Design review of the part built by this model. Coordinates are the model's own, in mm. A direction names the side the tool comes from. Give positions to 0.01 mm unless a question says otherwise; leave off trailing zeros. Order: outer loops, then holes, each group sorted by start corner. A loop starts at its lowest first (then second) coordinate and runs counter-clockwise, first axis right, second up. Notation, with made-up numbers: (83, 64.25) -> (127, 64.25) arc R8 ccw to (127, 75.25) -> close; hole circle Ø4 at (66, 2.25). An arc over 180 degrees is marked (long way). Answer in a Markdown table with one row per item. Add a question column.
```python
from build123d import *

# Parameters (mm, degrees)
BOSS_EXTRUDE1_DEPTH                                = 5.9944
FILLET1_R                                          = 1.5875
CSK_FOR_10_FLAT_HEAD_MACHINE_SCREW_100_D           = 5.1054
CSK_FOR_10_FLAT_HEAD_MACHINE_SCREW_100_CSINK_D     = 9.779
CSK_FOR_10_FLAT_HEAD_MACHINE_SCREW_100_CSINK_ANGLE = 100


with BuildPart() as part:
    # Sketch1 → Boss-Extrude1 (new body)
    with BuildSketch(Plane(origin=(0, 0, 0), x_dir=(1, 0, 0), z_dir=(0, 1, 0))):
        with BuildLine():
            Line((-35.898566824, -38.1), (35.898566824, -38.1))
            ThreePointArc((35.898566824, -38.1), (45.716712095, -35.375027517), (52.726020022, -27.9796875))
            ThreePointArc((52.726020022, -27.9796875), (59.69, 0), (52.726020022, 27.9796875))
            ThreePointArc((52.726020022, 27.9796875), (45.716712095, 35.375027517), (35.898566824, 38.1))
            Line((35.898566824, 38.1), (-35.898566824, 38.1))
            ThreePointArc((-35.898566824, 38.1), (-45.716712095, 35.375027517), (-52.726020022, 27.9796875))
            ThreePointArc((-52.726020022, 27.9796875), (-59.69, 0), (-52.726020022, -27.9796875))
            ThreePointArc((-52.726020022, -27.9796875), (-45.716712095, -35.375027517), (-35.898566824, -38.1))
        make_face()
    extrude(amount=BOSS_EXTRUDE1_DEPTH)

    # Sketch3 → Revolve1 (revolve)
    with BuildSketch(Plane.XY, mode=Mode.PRIVATE) as revolve1_sk:
        with BuildLine():
            Line((-29.9974, 5.9944), (0, 5.9944))
            Line((0, 5.9944), (0, 17.6022))
            ThreePointArc((0, 17.6022), (-11.253106327, 17.031245116), (-22.39063481, 15.324244597))
            ThreePointArc((-22.39063481, 15.324244597), (-27.854703555, 12.013305151), (-29.9974, 5.9944))
        make_face()
    revolve(revolve1_sk.sketch.rotate(Axis((0, 17.6022, 0), (0, -1, 0)), 180), axis=Axis((0, 17.6022, 0), (0, -1, 0)))

    # Fillet1
    fillet1_edges = [part.edges().sort_by_distance(p)[0] for p in [
        (-29.9974, 5.9944, 0),
    ]]
    fillet(fillet1_edges, radius=FILLET1_R)

    # CSK for #10 Flat Head Machine Screw (100)1 (through all)
    with Locations(Plane(origin=(0, 5.9944, 0), x_dir=(-1, 0, 0), z_dir=(0, 1, 0))):
        with Locations((41.91, -20.32), (41.91, 20.32), (-41.91, -20.32), (-41.91, 20.32)):
            CounterSinkHole(CSK_FOR_10_FLAT_HEAD_MACHINE_SCREW_100_D / 2, CSK_FOR_10_FLAT_HEAD_MACHINE_SCREW_100_CSINK_D / 2, counter_sink_angle=CSK_FOR_10_FLAT_HEAD_MACHINE_SCREW_100_CSINK_ANGLE)


solid = part.part
```
1) Add section C-C, the plane x = -34.5. Write out the cut boundary in (y, z), and give its area (3 significant figures).
2) Mouldability with a two-part tool opening along X and no side actions: class faces 3 (the face through (-44.03, 4.13, 18.7)), 4 (the face through (1, 3, -38.1)), 5 (the face through (45.84, 2.96, -35.3)) as +X half, -X half, draft (parallel to the pull), parting line (faces both ways), or undercut.
3) For L1, parallel to Z at x = -41.91, y = 3.15; L2, parallel to X at y = 2.7, z = -20.32; L3, parallel to Y at x = -24, z = 21, list the stretches that pass through material, from the lowest coordinate up.
4) Add section B-B, the plane z = 20.32. Give the number of separate pieces and of enclosed holes in the cut face, and give its area (3 significant figures).
5) Machinability: for faces 1 (the face through (59.69, 2.96, 0.41)), 2 (the face through (-27.4, 5.994, 16.4)), which of the approach directions +Z, -Z, +X, -X, +Y, -Y give a long, thin tool a straight path to every point of the face, cutting with its end or side? Answer none if there is none.
6) Add section A-A, the plane x = 41.91. Write out the cut boundary in (y, z).
7) Clearance check with flat-ended pins moving along their axes: P1, Ø3, axis at x = -41.91, z = -20.32, coming from the -Y side; P2, Ø1, axis at y = 13.5, z = -2.5, coming from the -X side; P3, Ø4, axis at y = 2, z = 2.5, coming from the -X side; P4, Ø4, axis at x = 16, y = 12, coming from the +Z side. State where each tip first meets the part, or that it passes through.
Verdict:
| question | item | result |
|---|---|---|
| 1 | outline | (0, -38.1) -> (5.99, -38.1) -> (5.99, 38.1) -> (0, 38.1) -> close |
| 1 | area | 457 mm2 |
| 2 | face 3 | undercut |
| 2 | face 4 | draft |
| 2 | face 5 | +X half |
| 3 | L1 | z = -37.13 to -22.87, -17.77 to 17.77, 22.87 to 37.13 |
| 3 | L2 | x = -56.12 to -44.46, -39.36 to 39.36, 44.46 to 56.12 |
| 3 | L3 | y = 0 to 5.99 |
| 4 | separate pieces | 3 |
| 4 | enclosed holes | 0 |
| 4 | area | 968 mm2 |
| 5 | face 1 | +X, +Y, -Y |
| 5 | face 2 | +Y |
| 6 | outline | (0, -37.13) -> (5.99, -37.13) -> (5.99, -25.21) -> (4.03, -22.87) -> (0, -22.87) -> close; (0, -17.77) -> (4.03, -17.77) -> (5.99, -15.43) -> (5.99, 15.43) -> (4.03, 17.77) -> (0, 17.77) -> close; (0, 22.87) -> (4.03, 22.87) -> (5.99, 25.21) -> (5.99, 37.13) -> (0, 37.13) -> close |
| 7 | P1 | passes through |
| 7 | P2 | stops at x = -26.81 |
| 7 | P3 | stops at x = -59.69 |
| 7 | P4 | stops at z = 24.86 |
